from build123d import *

# Parameters (mm, degrees)
SKIZZE1_R                       = 1.1
AUFSATZ_LINEAR_AUSTRAGEN1_DEPTH = 2.5


with BuildPart() as part:
    # Skizze1 → Aufsatz-Linear austragen1 (new body)
    with BuildSketch(Plane.XY):
        Polygon((-4, 12), (4, 12), (12, 4), (12, -4), (4, -12), (-4, -12), (-12, -4), (-12, 4), align=None)
        with Locations((-2, 10)):
            Circle(SKIZZE1_R, mode=Mode.SUBTRACT)
        with Locations((2, 6)):
            Circle(SKIZZE1_R, mode=Mode.SUBTRACT)
        with Locations((10, 2)):
            Circle(SKIZZE1_R, mode=Mode.SUBTRACT)
        with Locations((6, -2)):
            Circle(SKIZZE1_R, mode=Mode.SUBTRACT)
        with Locations((2, -10)):
            Circle(SKIZZE1_R, mode=Mode.SUBTRACT)
        with Locations((-2, -6)):
            Circle(SKIZZE1_R, mode=Mode.SUBTRACT)
        with Locations((-6, 2)):
            Circle(SKIZZE1_R, mode=Mode.SUBTRACT)
        with Locations((-10, -2)):
            Circle(SKIZZE1_R, mode=Mode.SUBTRACT)
        with Locations((-6, 6)):
            Circle(SKIZZE1_R, mode=Mode.SUBTRACT)
        with Locations((6, 6)):
            Circle(SKIZZE1_R, mode=Mode.SUBTRACT)
        with Locations((6, -6)):
            Circle(SKIZZE1_R, mode=Mode.SUBTRACT)
        with Locations((-6, -6)):
            Circle(SKIZZE1_R, mode=Mode.SUBTRACT)
    extrude(amount=AUFSATZ_LINEAR_AUSTRAGEN1_DEPTH)


solid = part.part
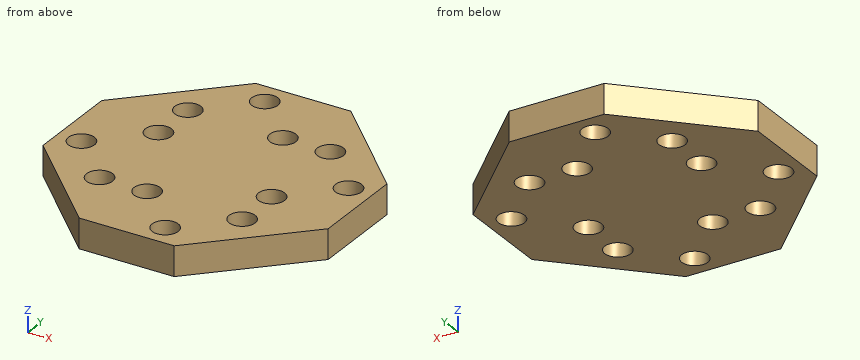
The model under review builds one solid part; all positions refer to its coordinate system, in mm. Coordinates: 2 decimals unless noted, no trailing zeros. Loops run counter-clockwise (first coordinate to the right, second up) from the corner with the lowest first, then second, coordinate; pieces in that order, holes last. Notation, with made-up numbers: (67, 55.5) -> (118, 55.5) arc R8 ccw to (118, 60.5) -> close; hole circle Ø6 at (-28, 86.5). An arc over 180 degrees is marked (long way). Use a Markdown table: item, result. Add a question column.
1. Add section A-A on y = -10. Write out the cut boundary in (x, z).
2. Add section D-D on y = 6. Write out the cut boundary in (x, z).
3. Add section B-B on x = 6. Write out the cut boundary in (y, z), plus the area to 3 significant figures.
4. Clearance check with flat-ended pins moving along their axes: pin 1 Ø2 at (x, y) = (-6, 2) entering from +Z; pin 2 Ø1.5 at (y, z) = (6.5, 0.5) entering from -X. State where each tip first meets the part, or that it passes through.
5. To check wall thickness, follow line 1 (Y direction, x = 2, z = 1.4); line 2 (X direction, y = 2.5, z = 1.2); line 3 (X direction, y = 5, z = 0.3). State the ranges of each line that lie inside material, in increasing order.
Returned:
| question | item | result |
|---|---|---|
| 1 | outline | (-6, 0) -> (0.9, 0) -> (0.9, 2.5) -> (-6, 2.5) -> close; (3.1, 0) -> (6, 0) -> (6, 2.5) -> (3.1, 2.5) -> close |
| 2 | outline | (-10, 0) -> (-7.1, 0) -> (-7.1, 2.5) -> (-10, 2.5) -> close; (-4.9, 0) -> (0.9, 0) -> (0.9, 2.5) -> (-4.9, 2.5) -> close; (3.1, 0) -> (4.9, 0) -> (4.9, 2.5) -> (3.1, 2.5) -> close; (7.1, 0) -> (10, 0) -> (10, 2.5) -> (7.1, 2.5) -> close |
| 3 | outline | (-10, 0) -> (-7.1, 0) -> (-7.1, 2.5) -> (-10, 2.5) -> close; (-4.9, 0) -> (-3.1, 0) -> (-3.1, 2.5) -> (-4.9, 2.5) -> close; (-0.9, 0) -> (4.9, 0) -> (4.9, 2.5) -> (-0.9, 2.5) -> close; (7.1, 0) -> (10, 0) -> (10, 2.5) -> (7.1, 2.5) -> close |
| 3 | area | 33.5 mm² |
| 4 | pin 1 | passes through |
| 4 | pin 2 | stops at x = -10.25 |
| 5 | line 1 | y = -12 to -11.1, -8.9 to 4.9, 7.1 to 12 |
| 5 | line 2 | x = -12 to -6.98, -5.02 to 9.02, 10.98 to 12 |
| 5 | line 3 | x = -11 to -6.46, -5.54 to 1.54, 2.46 to 5.54, 6.46 to 11 |
